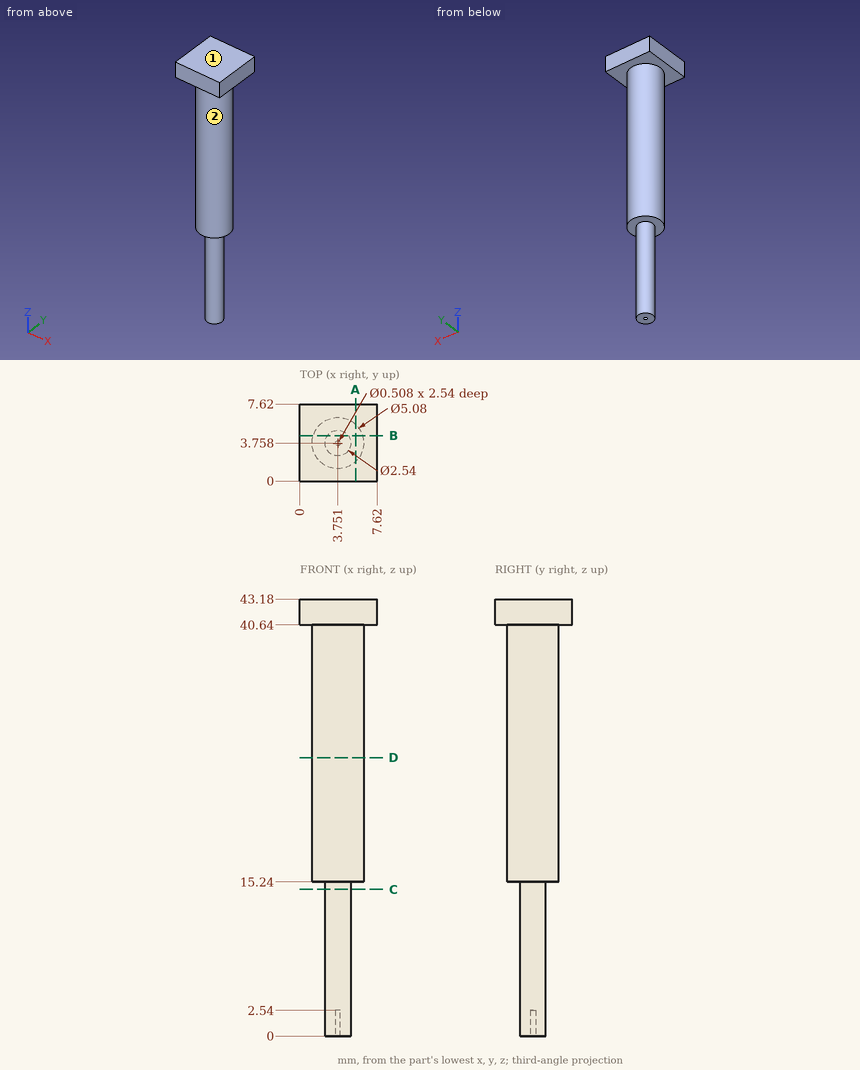
Input: dimensioned drawing with shaded views. Units: mm. Origin: part minimum x, y, z. A direction names the side the tool comes from. Give positions to 0.01 mm unless a question says otherwise; leave off trailing zeros. Loops run counter-clockwise (first coordinate to the right, second up) from the corner with the lowest first, then second, coordinate; pieces in that order, holes last. Notation, with made-up numbers: (16.5, -23.5) -> (64.5, -23.5) arc R21 ccw to (64.5, 12.5) -> close; hole circle Ø7 at (42.25, -35.75). An arc over 180 degrees is marked (long way). Use a Markdown table: item, result. Add a question column.
1) First-contact query: pin 1 (4 mm diameter, centred on x = 4, z = 22, fed in from -Y); pin 2 (2 mm diameter, centred on y = 1.5, z = 26, fed in from +X); pin 3 (2 mm diameter, centred on x = 5.5, z = 8.5, fed in from +Y). Flat tips, straight axial feed; report the tip coordinate or a pass-through.
2) Line query: line 1 along Z through (x, y) = (5, 6); line 2 along Y through (x, z) = (3.75, 20.5); line 3 along Z through (x, y) = (1.75, 3.25). Output: solid intervals per line, ascending. Write a range as [from, to].
3) Section query B-B, the plane y = 4.5. Return the cut outline in (x, z).
4) Section query C-C, the plane z = 14.5. Return the cut outline in (x, y).
5) Reachability of the marked faces 1 and 2 from +Z, -Z, +X, -X, +Y, -Y: full face, straight path, thin tool, end or side. Return the list, or none.
6) Section query A-A, the plane x = 5.5. Return the cut outline in (y, z), then the cut area to 3 significant figures.
7) Section query D-D, the plane z = 27.5. Return the cut outline in (x, y), then the cut area to 3 significant figures.
Numbers:
| question | item | result |
|---|---|---|
| 1 | pin 1 | stops at y = 1.22 |
| 1 | pin 2 | stops at x = 5.96 |
| 1 | pin 3 | stops at y = 4.78 |
| 2 | line 1 | z = [40.64, 43.18] |
| 2 | line 2 | y = [1.22, 6.3] |
| 2 | line 3 | z = [15.24, 43.18] |
| 3 | outline | (0, 40.64) -> (1.32, 40.64) -> (1.32, 15.24) -> (2.72, 15.24) -> (2.72, 0) -> (4.78, 0) -> (4.78, 15.24) -> (6.18, 15.24) -> (6.18, 40.64) -> (7.62, 40.64) -> (7.62, 43.18) -> (0, 43.18) -> close |
| 4 | outline | circle Ø2.54 at (3.75, 3.76) |
| 5 | face 1 | +Z, +X, -X, +Y, -Y |
| 5 | face 2 | -Z |
| 6 | outline | (0, 40.64) -> (1.92, 40.64) -> (1.92, 15.24) -> (5.6, 15.24) -> (5.6, 40.64) -> (7.62, 40.64) -> (7.62, 43.18) -> (0, 43.18) -> close |
| 6 | area | 113 mm2 |
| 7 | outline | circle Ø5.08 at (3.75, 3.76) |
| 7 | area | 20.3 mm2 |
